```python
from build123d import *

# Parameters (mm, degrees)
SKETCH1_W           = 58
SKETCH1_H           = 46
BOSS_EXTRUDE1_DEPTH = 4.5
SKETCH2_W           = 55.1
SKETCH2_H           = 43.1
SKETCH2_W_2         = 53.1
SKETCH2_H_2         = 41.1
BOSS_EXTRUDE2_DEPTH = 2
SKETCH3_W           = 53.1
SKETCH3_H           = 41.1
CUT_EXTRUDE1_DEPTH  = 3
SKETCH4_W           = 1
SKETCH4_H           = 15.5
CUT_EXTRUDE2_DEPTH  = 2
CUT_EXTRUDE4_START  = 5
SKETCH5_W           = 54.1
SKETCH5_H           = 1
CUT_EXTRUDE4_DEPTH  = 2
FILLET1_R           = 2
SKETCH6_W           = 1.45
SKETCH6_H           = 14.95
CUT_EXTRUDE5_DEPTH  = 5.5


with BuildPart() as part:
    # Sketch1 → Boss-Extrude1 (new body)
    with BuildSketch(Plane(origin=(0, 0, 0), x_dir=(1, 0, 0), z_dir=(0, 1, 0))):
        with Locations((2.929896907, -5.540206186)):
            Rectangle(SKETCH1_W, SKETCH1_H)
    extrude(amount=BOSS_EXTRUDE1_DEPTH)

    # Sketch2 → Boss-Extrude2 (add)
    with BuildSketch(Plane(origin=(0, 4.5, 0), x_dir=(1, 0, 0), z_dir=(0, 1, 0))):
        with Locations((2.929896907, -5.540206186)):
            Rectangle(SKETCH2_W, SKETCH2_H)
        with Locations((2.929896907, -5.540206186)):
            Rectangle(SKETCH2_W_2, SKETCH2_H_2, mode=Mode.SUBTRACT)
    extrude(amount=BOSS_EXTRUDE2_DEPTH)

    # Sketch3 → Cut-Extrude1 (cut)
    with BuildSketch(Plane(origin=(0, 4.5, 0), x_dir=(1, 0, 0), z_dir=(0, 1, 0))):
        with Locations((2.929896907, -5.540206186)):
            Rectangle(SKETCH3_W, SKETCH3_H)
    extrude(amount=-CUT_EXTRUDE1_DEPTH, mode=Mode.SUBTRACT)

    # Sketch4 → Cut-Extrude2 (cut)
    with BuildSketch(Plane(origin=(0, 6.5, 0), x_dir=(1, 0, 0), z_dir=(0, 1, 0))):
        with Locations((29.979896907, -19.340206186)):
            Rectangle(SKETCH4_W, SKETCH4_H)
    extrude(amount=-CUT_EXTRUDE2_DEPTH, mode=Mode.SUBTRACT)

    # Sketch5 → Cut-Extrude4 (cut)
    with BuildSketch(Plane(origin=(0, 1.5, 0), x_dir=(1, 0, 0), z_dir=(0, 1, 0)).offset(CUT_EXTRUDE4_START)):
        with Locations((2.429896907, -26.590206186)):
            Rectangle(SKETCH5_W, SKETCH5_H)
    extrude(amount=-CUT_EXTRUDE4_DEPTH, mode=Mode.SUBTRACT)

    # Fillet1
    fillet1_edges = [part.edges().sort_by_distance(p)[0] for p in [
        (-26.070103093, 2.25, -17.459793814),
        (31.929896907, 2.25, -17.459793814),
        (31.929896907, 2.25, 28.540206186),
        (-26.070103093, 2.25, 28.540206186),
    ]]
    fillet(fillet1_edges, radius=FILLET1_R)

    # Sketch6 → Cut-Extrude5 (cut, through all)
    with BuildSketch(Plane(origin=(0, 4.5, 0), x_dir=(1, 0, 0), z_dir=(0, 1, 0))):
        with Locations((31.204896907, -19.065206186)):
            Rectangle(SKETCH6_W, SKETCH6_H)
    extrude(amount=-CUT_EXTRUDE5_DEPTH, mode=Mode.SUBTRACT)


solid = part.part
```
Could you check a few things on this model? Use its own coordinates, in mm. A direction names the side the tool comes from. Coordinates: 2 decimals unless noted, no trailing zeros. Write each loop counter-clockwise with the first axis right and the second up, starting at its lowest first coordinate (ties: lowest second). Pieces come first, ordered by that corner, then holes. Notation, with made-up numbers: (2.5, 12.25) -> (14.5, 12.25) arc R5 cw to (14.5, 18.25) -> close; hole circle Ø10 at (29, -28). An arc over 180 degrees is marked (long way). Write item = value, one per line. Start each with the question number.
(1) Will these pins go through, and if not, where does the flat tip stop? pin 1 (1.5 mm diameter, centred on y = 5, z = 15, fed in from +X); pin 2 (14 mm diameter, centred on x = -9.5, z = 5.5, fed in from +Y); pin 3 (0.6 mm diameter, centred on y = 5, z = 14, fed in from -X).
(2) Which directions (+Z, -Z, +X, -X, +Y, -Y) give clear straight access to the entire face, cutting with the end or side of a thin tool? Please do faces 1 (the face through (3, 4, -15.01)), 2 (the face through (3, 5, -16.01)), 3 (the face through (31, 2, 11.59)), 4 (the face through (30.48, 5, -2)).
(3) I want a section at C-C (z = -10). Please give me the cut outline in (x, y).
(4) I want a section at B-B (y = 3.25). Please give me the cut outline in (x, z), plus the area to 3 significant figures.
(5) I want a section at D-D (z = 19). Please give me the cut outline in (x, y), plus the area to 3 significant figures.
(6) I need wall thicknesses on line 1 (X direction, y = 3.25, z = -3.5); line 2 (X direction, y = 5.5, z = 8.5); line 3 (Z direction, x = -8.5, y = 2). Which ranges of each line are inside material? Lowest first, please. Write a range as [from, to].
(7) We'd pull the mould along Z, two halves only. Please class faces 5 (the face through (31, 2, 26.54)), 6 (the face through (3, 1.5, 5)), 7 (the face through (31.33, 2.28, 27.97)), 8 (the face through (-24.62, 5, 5)): released by +Z, released by -Z, zero draft, split by the parting line, or undercut.
(8) I want a section at A-A (x = 10). Please give me the cut outline in (y, z), plus the area to 3 significant figures.
Result set:
q1.pin_1 = 30.48
q1.pin_2 = 1.5
q1.pin_3 = -24.62
q2.face_1 = +Y
q2.face_2 = -Z, +X, -X, +Y
q2.face_3 = +X, +Y, -Y
q2.face_4 = +Z, -Z, +X, +Y
q3.outline = (-26.07, 0) -> (31.93, 0) -> (31.93, 4.5) -> (30.48, 4.5) -> (30.48, 6.5) -> (29.48, 6.5) -> (29.48, 1.5) -> (-23.62, 1.5) -> (-23.62, 6.5) -> (-24.62, 6.5) -> (-24.62, 4.5) -> (-26.07, 4.5) -> close
q4.outline = (-26.07, -15.46) arc R2 ccw to (-24.07, -17.46) -> (29.93, -17.46) arc R2 ccw to (31.93, -15.46) -> (31.93, 11.59) -> (30.48, 11.59) -> (30.48, 26.54) -> (31.93, 26.54) arc R2 ccw to (29.93, 28.54) -> (-24.07, 28.54) arc R2 ccw to (-26.07, 26.54) -> close; hole (-23.62, -15.01) -> (29.48, -15.01) -> (29.48, 26.09) -> (-23.62, 26.09) -> close
q4.area = 460 mm2
q5.outline = (-26.07, 0) -> (30.48, 0) -> (30.48, 4.5) -> (29.48, 4.5) -> (29.48, 1.5) -> (-23.62, 1.5) -> (-23.62, 6.5) -> (-24.62, 6.5) -> (-24.62, 4.5) -> (-26.07, 4.5) -> close
q5.area = 97.2 mm2
q6.line_1 = [-26.07, -23.62], [29.48, 31.93]
q6.line_2 = [-24.62, -23.62], [29.48, 30.48]
q6.line_3 = [-17.46, -15.01], [26.09, 28.54]
q7.face_5 = undercut
q7.face_6 = undercut
q7.face_7 = released by +Z
q7.face_8 = zero draft
q8.outline = (0, -17.46) -> (4.5, -17.46) -> (4.5, -16.01) -> (6.5, -16.01) -> (6.5, -15.01) -> (1.5, -15.01) -> (1.5, 26.09) -> (4.5, 26.09) -> (4.5, 28.54) -> (0, 28.54) -> close
q8.area = 85.7 mm2
